Design review of the part shown in the three views and the two pictorial views. Dimensions are in mm from the part's minimum x, y and z. A direction names the side the tool comes from. Give positions to 0.01 mm unless a question says otherwise; leave off trailing zeros. Loops run counter-clockwise (first coordinate to the right, second up) from the corner with the lowest first, then second, coordinate; pieces in that order, holes last. Notation, with made-up numbers: (70, -32) - (110, -32) arc R12 ccw to (110, -9) - close; hole circle Ø10 at (2.25, -4). An arc over 180 degrees is marked (long way). Return JSON: item names as keys, results as strings. Group by question number.
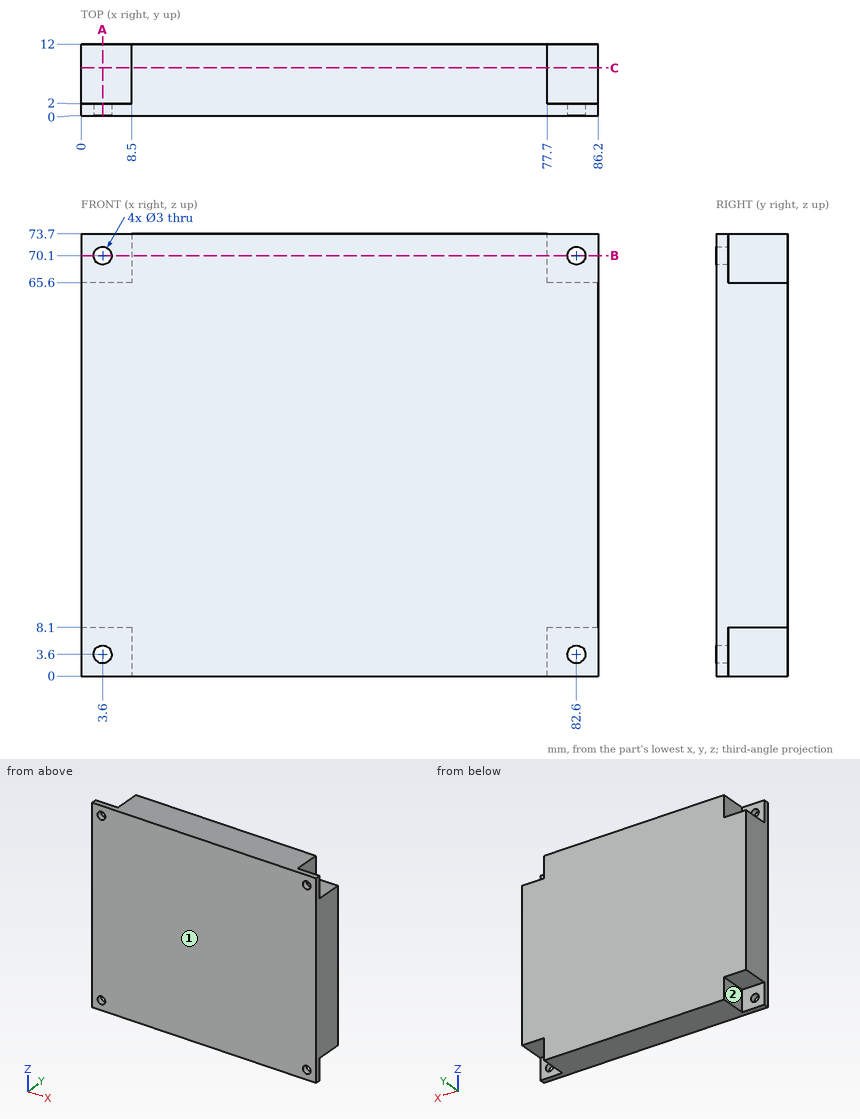
Item 1: For L1, parallel to X at y = 0.75, z = 70.1; L2, parallel to Z at x = 80.5, y = 11.5, list the stretches that pass through material, from the lowest coordinate up. Write a range as from..to.
Item 2: For P1, Ø1.8, axis at x = 3.6, z = 3.6, coming from the +Y side; P2, Ø7, axis at x = 81.5, y = 8.5, coming from the -Z side; P3, Ø4, axis at x = 82.6, z = 3.6, coming from the +Y side; P4, Ø4, axis at y = 6, z = 69.5, coming from the -X side, all flat-tipped, find the tip position at first contact; note any pin that passes through.
Item 3: Take a section at B-B (z = 70.1). State the section outline as (x, y) points, then the cut area to 3 significant figures.
Item 4: Take a section at C-C (y = 8). State the section outline as (x, z) points, then the cut area to 3 significant figures.
Item 5: Take a section at A-A (x = 3.6). State the section outline as (y, z) points, then the cut area to 3 significant figures.
Item 6: Tool access review of the marked faces 1 and 2: name each direction out of +Z, -Z, +X, -X, +Y, -Y from which nothing blocks a thin tool from reaching the whole face with its end or side.
Check sheet entries:
{
 "1": {"L1": "x = 0..2.1, 5.1..81.1, 84.1..86.2", "L2": "z = 8.1..65.6"},
 "2": {"P1": "passes through", "P2": "stops at z = 8.1", "P3": "stops at y = 2", "P4": "stops at x = 8.5"},
 "3": {"outline": "(0, 0) - (2.1, 0) - (2.1, 2) - (0, 2) - close; (5.1, 0) - (81.1, 0) - (81.1, 2) - (77.7, 2) - (77.7, 12) - (8.5, 12) - (8.5, 2) - (5.1, 2) - close; (84.1, 0) - (86.2, 0) - (86.2, 2) - (84.1, 2) - close", "area": "852 mm^2"},
 "4": {"outline": "(0, 8.1) - (8.5, 8.1) - (8.5, 0) - (77.7, 0) - (77.7, 8.1) - (86.2, 8.1) - (86.2, 65.6) - (77.7, 65.6) - (77.7, 73.7) - (8.5, 73.7) - (8.5, 65.6) - (0, 65.6) - close", "area": "6,080 mm^2"},
 "5": {"outline": "(0, 0) - (2, 0) - (2, 2.1) - (0, 2.1) - close; (0, 5.1) - (2, 5.1) - (2, 8.1) - (12, 8.1) - (12, 65.6) - (2, 65.6) - (2, 68.6) - (0, 68.6) - close; (0, 71.6) - (2, 71.6) - (2, 73.7) - (0, 73.7) - close", "area": "710 mm^2"},
 "6": {"face 1": "+Z, -Z, +X, -X, -Y", "face 2": "-Z, -X, +Y"}
}
